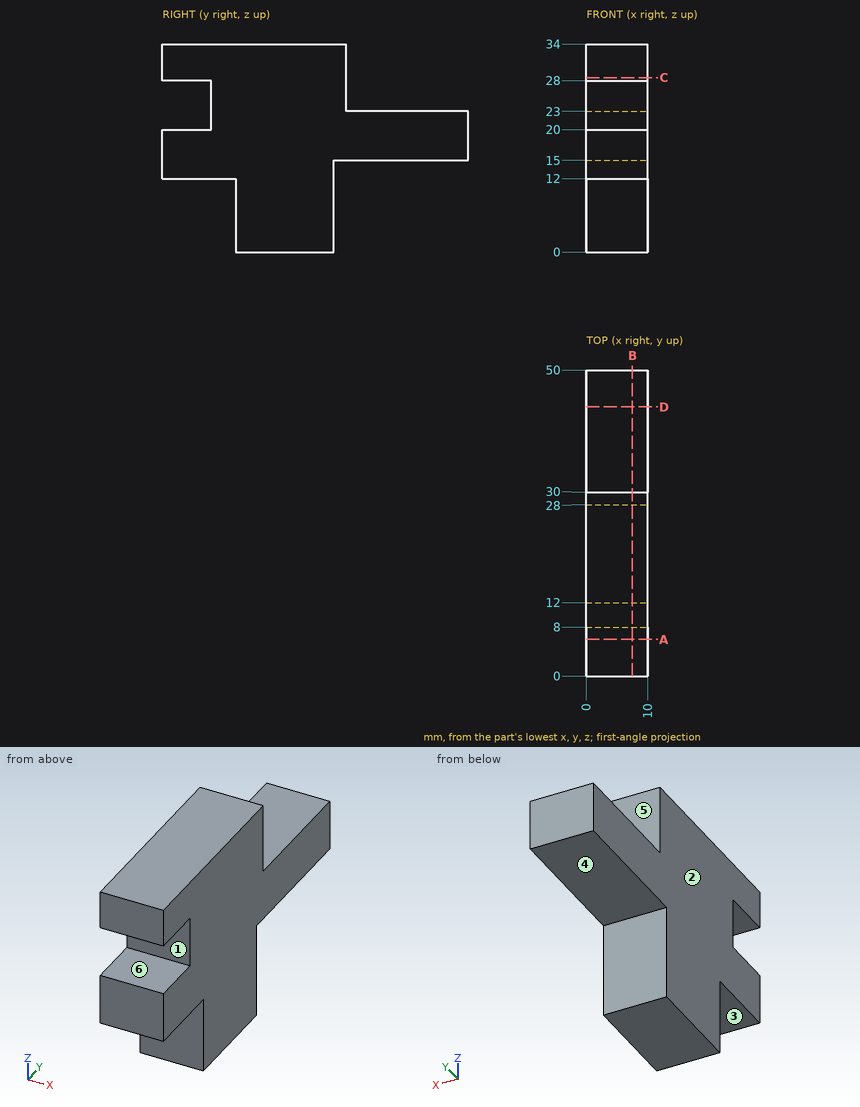
Drawing for the job (mm, zero at the part's lowest x, y, z). A direction names the side the tool comes from. Round coordinates to 2 decimals unless told otherwise and drop trailing zeros. Loops run counter-clockwise (first coordinate to the right, second up) from the corner with the lowest first, then second, coordinate; pieces in that order, holes last.
1. Band-saw the part on D-D, the plane y = 44. List the corners of the cut face in (x, z), and give its area (3 significant figures).
Check values:
outline: (0, 15) - (10, 15) - (10, 23) - (0, 23) - close
area: 80.0 mm2
2. Band-saw the part on A-A, the plane y = 6. List the corners of the cut face in (x, z).
Check values:
outline: (0, 12) - (10, 12) - (10, 20) - (0, 20) - close; (0, 28) - (10, 28) - (10, 34) - (0, 34) - close
3. Band-saw the part on B-B, the plane x = 7.5. List the corners of the cut face in (y, z), and give its area (3 significant figures).
Check values:
outline: (0, 12) - (12, 12) - (12, 0) - (28, 0) - (28, 15) - (50, 15) - (50, 23) - (30, 23) - (30, 34) - (0, 34) - (0, 28) - (8, 28) - (8, 20) - (0, 20) - close
area: 942 mm2
4. Tool access for the marked faces 4, 5 and 6: list every direction of +Z, -Z, +X, -X, +Y, -Y with a clear straight run to the whole face (end or side of a thin tool).
Check values:
face 4: -Z, +X, -X, +Y
face 5: +Z, +X, -X, +Y
face 6: +X, -X, -Y
5. Band-saw the part on C-C, the plane z = 28.5. List the corners of the cut face in (x, y), and give its area (3 significant figures).
Check values:
outline: (0, 0) - (10, 0) - (10, 30) - (0, 30) - close
area: 300 mm2
6. Drop a flat-ended pin along its axis: P1, Ø5, axis at x = 4.5, z = 9.5, coming from the +Y side. Give the stop position or say it passes through.
Check values:
P1: stops at y = 28
7. Mould opens along Z. For the marked faces 1, 2 and 3 say: +Z half, -Z half, draft (parallel to the pull), parting line (faces both ways), or undercut.
Check values:
face 1: undercut
face 2: draft
face 3: -Z half
8. Wall check: probe 1 along Y at (x, z) = (8.25, 6.5); probe 2 along Y at (x, z) = (2.25, 14.5); probe 3 along Z at (x, y) = (7.75, 38.5). Give the ranges that are in metal, low to high.
Check values:
probe 1: y = 12 to 28
probe 2: y = 0 to 28
probe 3: z = 15 to 23
